Geometry: final body of the model. Coordinates: model frame, mm. Face numbers are marked on the shaded views. A direction names the side the tool comes from. Give positions to 0.01 mm unless a question says otherwise; leave off trailing zeros. Loops run counter-clockwise (first coordinate to the right, second up) from the corner with the lowest first, then second, coordinate; pieces in that order, holes last. Notation, with made-up numbers: (-35, 50.5) -> (-30, 50.5) arc R21 cw to (-30, 73.5) -> close; hole circle Ø8 at (71, 4). An arc over 180 degrees is marked (long way). Answer in a Markdown table with one row per item. Add a question column.
1) Access query for the marked faces 1, 2, 3 and 4. Directions: +Z, -Z, +X, -X, +Y, -Y. A direction counts if a zero-diameter tool reaches every point of the face in a straight line with its end or side. Return the directions, or none.
2) Line query: line 1 (Y direction, x = -5, z = 116); line 2 (Y direction, x = 9, z = 141); line 3 (X direction, y = 0.5, z = 87). Output: solid intervals per line, ascending. Write a range as from..to.
3) Section query A-A (z = 124). Return the cut outline in (x, y), plus the area to 3 significant figures.
4) Section query B-B (x = 0). Return the cut outline in (y, z), plus the area to 3 significant figures.
5) First-contact query: P1, Ø18, axis at y = -13.5, z = 162.5, coming from the +X side; P2, Ø4, axis at y = -72.5, z = 135, coming from the -X side; P3, Ø13.5, axis at x = 0, z = 155, coming from the +Y side. Flat tips, straight axial feed; report the tip coordinate or a pass-through.
6) Section query D-D (z = 104.5). Return the cut outline in (x, y).
7) Section query C-C (y = -16.5). Return the cut outline in (x, z), plus the area to 3 significant figures.
8) Draft query along Y for the marked faces 5, 6, 7 and 8. Return one class per face: +Y half, -Y half, draft (parallel to the pull), parting line (faces both ways), or undercut.
```python
from build123d import *

# Parameters (mm, degrees)
F0_R     = 53.51649
F1_DEPTH = 115.161
F2_W     = 44.614081
F2_H     = 18.834734
F2_W_2   = 53.55269
F2_H_2   = 35.868514
F3_DEPTH = 68.41306
F4_R     = 18.843136
F5_DEPTH = 66.90822


with BuildPart() as f1:
    # F0 (on Top) → F1 (new body)
    with BuildSketch(Plane.XY):
        Circle(F0_R)
    extrude(amount=F1_DEPTH)

    # F2 (on face) → F3 (join)
    with BuildSketch(Plane.XY.offset(115.161)):
        with Locations((-6.069197, 28.253733)):
            Rectangle(F2_W, F2_H)
        with Locations((0, -17.934257)):
            Rectangle(F2_W_2, F2_H_2)
    extrude(amount=F3_DEPTH)

    # F4 (on face) → F5 (join)
    with BuildSketch(Plane.XZ.offset(35.868514)):
        with Locations((0, 152.677178)):
            Circle(F4_R)
    extrude(amount=F5_DEPTH)


solid = f1.part
```
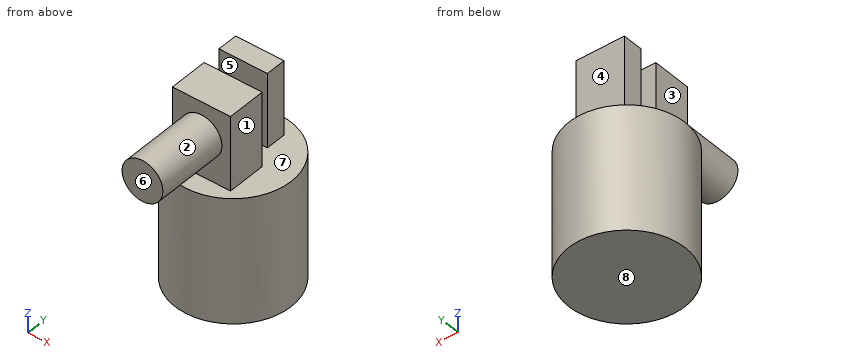
Evaluation:
| question | item | result |
|---|---|---|
| 1 | face 1 | +Z, +X, +Y, -Y |
| 1 | face 2 | -Y |
| 1 | face 3 | +Z, -X, -Y |
| 1 | face 4 | +Z, +X, -X, +Y |
| 2 | line 1 | -35.87..0, 18.84..37.67 |
| 2 | line 2 | -102.78..0, 18.84..37.67 |
| 2 | line 3 | -53.51..53.51 |
| 3 | outline | (-28.38, 18.84) -> (16.24, 18.84) -> (16.24, 37.67) -> (-28.38, 37.67) -> close; (-26.78, -35.87) -> (26.78, -35.87) -> (26.78, 0) -> (-26.78, 0) -> close |
| 3 | area | 2,760 mm² |
| 4 | outline | (-102.78, 133.83) -> (-35.87, 133.83) -> (-35.87, 115.16) -> (-53.52, 115.16) -> (-53.52, 0) -> (53.52, 0) -> (53.52, 115.16) -> (37.67, 115.16) -> (37.67, 183.57) -> (18.84, 183.57) -> (18.84, 115.16) -> (0, 115.16) -> (0, 183.57) -> (-35.87, 183.57) -> (-35.87, 171.52) -> (-102.78, 171.52) -> close |
| 4 | area | 18,600 mm² |
| 5 | P1 | x = 26.78 |
| 5 | P2 | x = -10.45 |
| 5 | P3 | y = 37.67 |
| 6 | outline | circle Ø107.03 at (0, 0) |
| 7 | outline | (-50.91, 0) -> (50.91, 0) -> (50.91, 115.16) -> (26.78, 115.16) -> (26.78, 183.57) -> (-26.78, 183.57) -> (-26.78, 115.16) -> (-50.91, 115.16) -> close |
| 7 | area | 15,400 mm² |
| 8 | face 5 | undercut |
| 8 | face 6 | -Y half |
| 8 | face 7 | undercut |
| 8 | face 8 | draft |
